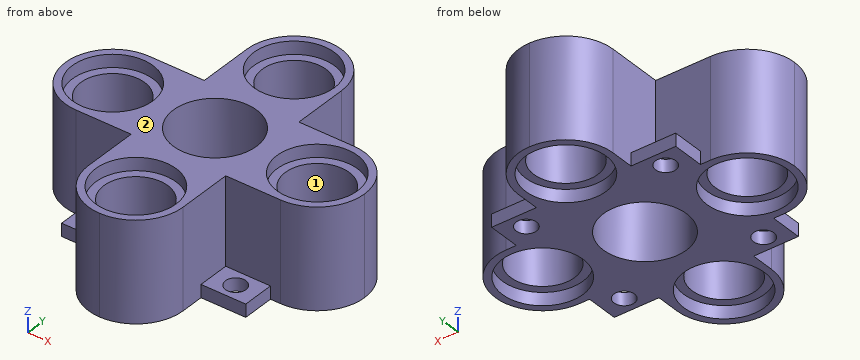
```python
from build123d import *

# Parameters (mm, degrees)
SKETCH_2_W          = 23.4
SKETCH_2_H          = 7.4
SKETCH_2_W_2        = 7.4
SKETCH_2_H_2        = 23.4
EXTRUDE_1_DEPTH     = 7.8
SKETCH_3_W          = 14.4
SKETCH_3_H          = 12.4
EXTRUDE_2_DEPTH     = 1
SKETCH_2_6_R        = 2.5
SKETCH_2_6_R_2      = 3.25
CUT_EXTRUDE_3_DEPTH = 19.292621463
SKETCH_2_3_R        = 3.15
CUT_EXTRUDE_1_DEPTH = 1
CUT_EXTRUDE_START   = 6.8
SKETCH_2_5_R        = 3.15
CUT_EXTRUDE_2_DEPTH = 1
SKETCH_4_R          = 0.8
CUT_EXTRUDE_4_DEPTH = 18.889102828


with BuildPart() as part:
    # 草图2 → 凸台-拉伸1 (new body)
    with BuildSketch(Plane.XY):
        Rectangle(SKETCH_2_W, SKETCH_2_H)
        Rectangle(SKETCH_2_W_2, SKETCH_2_H_2)
    extrude(amount=EXTRUDE_1_DEPTH)

    # 草图3 → 凸台-拉伸2 (add)
    with BuildSketch(Plane(origin=(0, 0, 0), x_dir=(-1, 0, 0), z_dir=(0, 0, -1))):
        Rectangle(SKETCH_3_W, SKETCH_3_H)
    extrude(amount=-EXTRUDE_2_DEPTH)

    # 草图2<6> → 切除-拉伸3 (cut, through all)
    with BuildSketch(Plane.XY):
        with BuildLine():
            Line((-3.7, 11.7), (-3.7, 8))
            ThreePointArc((-3.7, 8), (-2.61629509, 10.61629509), (0, 11.7))
            Line((0, 11.7), (-3.7, 11.7))
        make_face()
        with BuildLine():
            ThreePointArc((0, 11.7), (2.61629509, 10.61629509), (3.7, 8))
            Line((3.7, 8), (3.7, 11.7))
            Line((3.7, 11.7), (0, 11.7))
        make_face()
        with BuildLine():
            Line((11.7, 3.7), (8.000000006, 3.7))
            ThreePointArc((8.000000006, 3.7), (10.616295093, 2.616295088), (11.7, 0))
            Line((11.7, 0), (11.7, 3.7))
        make_face()
        with BuildLine():
            ThreePointArc((11.7, 0), (10.616295085, -2.616295096), (7.999999984, -3.7))
            Line((7.999999984, -3.7), (11.7, -3.7))
            Line((11.7, -3.7), (11.7, 0))
        make_face()
        with BuildLine():
            Line((3.7, -11.7), (3.7, -8))
            ThreePointArc((3.7, -8), (2.61629509, -10.61629509), (0, -11.7))
            Line((0, -11.7), (3.7, -11.7))
        make_face()
        with BuildLine():
            ThreePointArc((0, -11.7), (-2.616295094, -10.616295087), (-3.7, -7.99999999))
            Line((-3.7, -7.99999999), (-3.7, -11.7))
            Line((-3.7, -11.7), (0, -11.7))
        make_face()
        with BuildLine():
            Line((-11.7, -1.1e-08), (-11.7, -3.7))
            Line((-11.7, -3.7), (-8.000000004, -3.7))
            ThreePointArc((-8.000000004, -3.7), (-10.616295088, -2.616295093), (-11.7, -1.1e-08))
        make_face()
        with BuildLine():
            Line((-11.7, 3.7), (-11.7, -1.1e-08))
            ThreePointArc((-11.7, -1.1e-08), (-10.616295094, 2.616295086), (-8, 3.7))
            Line((-8, 3.7), (-11.7, 3.7))
        make_face()
        with Locations((0, 8)):
            Circle(SKETCH_2_6_R)
        with Locations((-8, 0)):
            Circle(SKETCH_2_6_R)
        Circle(SKETCH_2_6_R_2)
        with Locations((8, 0)):
            Circle(SKETCH_2_6_R)
        with Locations((0, -8)):
            Circle(SKETCH_2_6_R)
    extrude(amount=CUT_EXTRUDE_3_DEPTH, mode=Mode.SUBTRACT)

    # 草图2<3> → 切除-拉伸1 (cut)
    with BuildSketch(Plane.XY):
        with Locations((8, 0)):
            Circle(SKETCH_2_3_R)
        with Locations((-8, 0)):
            Circle(SKETCH_2_3_R)
        with Locations((0, 8)):
            Circle(SKETCH_2_3_R)
        with Locations((0, -8)):
            Circle(SKETCH_2_3_R)
    extrude(amount=CUT_EXTRUDE_1_DEPTH, mode=Mode.SUBTRACT)

    # 草图2<5> → 切除-拉伸2 (cut)
    with BuildSketch(Plane.XY.offset(CUT_EXTRUDE_START)):
        with Locations((8, 0)):
            Circle(SKETCH_2_5_R)
        with Locations((-8, 0)):
            Circle(SKETCH_2_5_R)
        with Locations((0, 8)):
            Circle(SKETCH_2_5_R)
        with Locations((0, -8)):
            Circle(SKETCH_2_5_R)
    extrude(amount=CUT_EXTRUDE_2_DEPTH, mode=Mode.SUBTRACT)

    # 草图4 → 切除-拉伸4 (cut, through all)
    with BuildSketch(Plane.XY.offset(1)):
        with Locations((-5.45, 4.95)):
            Circle(SKETCH_4_R)
        with Locations((5.45, 4.95)):
            Circle(SKETCH_4_R)
        with Locations((-5.45, -4.95)):
            Circle(SKETCH_4_R)
        with Locations((5.45, -4.95)):
            Circle(SKETCH_4_R)
    extrude(amount=-CUT_EXTRUDE_4_DEPTH, mode=Mode.SUBTRACT)


solid = part.part
```
Design review of the part built by this model. Coordinates are the model's own, in mm. Face numbers are marked on the shaded views. Coordinates: 2 decimals unless noted, no trailing zeros. Write each loop counter-clockwise with the first axis right and the second up, starting at its lowest first coordinate (ties: lowest second). Pieces come first, ordered by that corner, then holes.
1) To check wall thickness, follow L1, parallel to X at y = -2.5, z = 7; L2, parallel to Y at x = -4.75, z = 5.25; L3, parallel to X at y = -9, z = 2. State the ranges of each line that lie inside material, in increasing order.
2) Mouldability with a two-part tool opening along X and no side actions: class the marked faces 1 and 2 as +X half, -X half, draft (parallel to the pull), parting line (faces both ways), or undercut.
3) Add section B-B (y = -1.25). State how many separate pieces and enclosed holes the cut face has, plus the area to 3 significant figures.
4) Insertion check: pin 1 (1.3 mm diameter, centred on x = -6.5, z = 2.5, fed in from -Y); pin 2 (3.5 mm diameter, centred on x = 6, z = 4.5, fed in from +Y); pin 3 (3 mm diameter, centred on x = 0.5, y = -9, fed in from -Z). Each pin has a flat end and moves straight along its axis. Give the tip position at first contact, or say it passes through.
5) Add section A-A (z = 7.25). Write out the cut boundary in (x, y), plus the area to 3 significant figures.
Check result:
1. L1: x = -10.73 to -9.92, -6.08 to -2.08, 2.08 to 6.08, 9.92 to 10.73
1. L2: y = -3.7 to 3.7
1. L3: x = -3.56 to -2.29, 2.29 to 3.56
2. face 1: undercut
2. face 2: draft
3. separate pieces: 4
3. enclosed holes: 0
3. area: 59.0 mm2
4. pin 1: stops at y = -3.7
4. pin 2: stops at y = 3.7
4. pin 3: stops at z = 1
5. outline: (-8, -3.7) - (-3.7, -3.7) - (-3.7, -8) arc R3.7 ccw to (3.7, -8) - (3.7, -3.7) - (8, -3.7) arc R3.7 ccw to (8, 3.7) - (3.7, 3.7) - (3.7, 8) arc R3.7 ccw to (-3.7, 8) - (-3.7, 3.7) - (-8, 3.7) arc R3.7 ccw to start; hole circle Ø6.3 at (-8, 0); hole circle Ø6.5 at (0, 0); hole circle Ø6.3 at (0, -8); hole circle Ø6.3 at (0, 8); hole circle Ø6.3 at (8, 0)
5. area: 110 mm2
